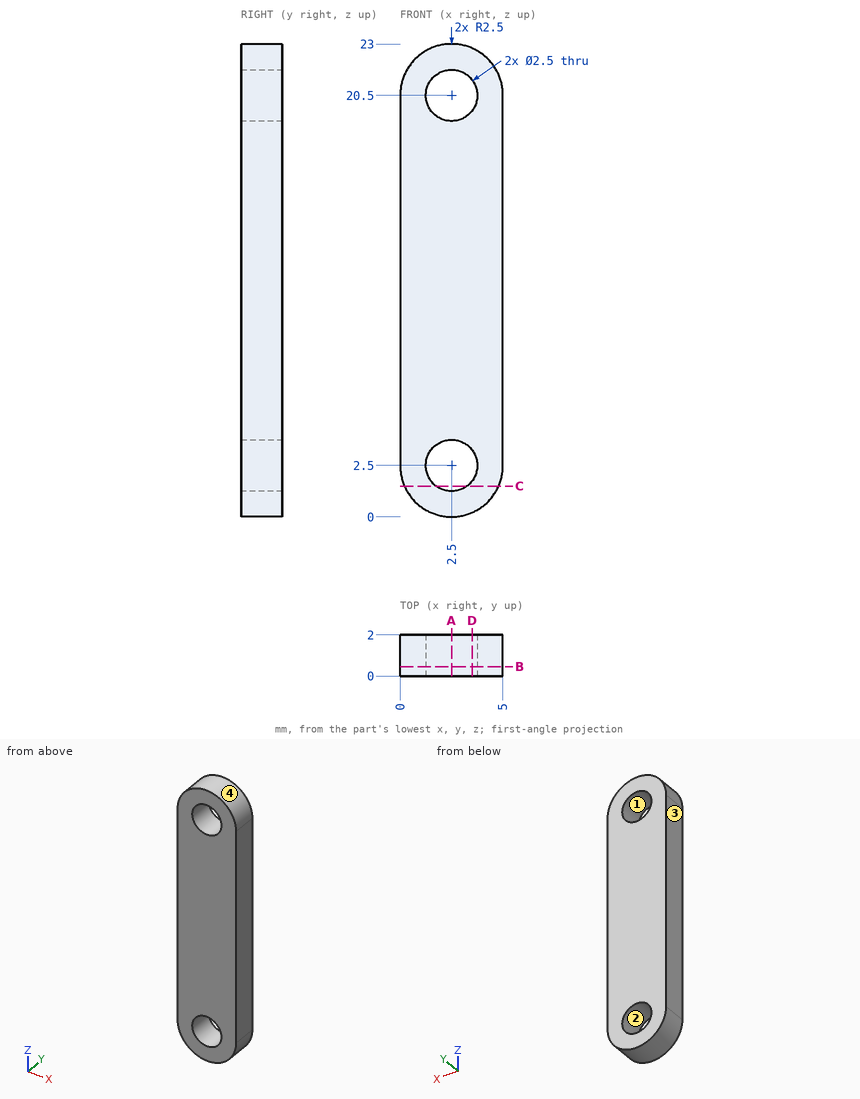
Geometry: see drawing. Coordinates: mm, zero at the bounding-box minimum. Give positions to 0.01 mm unless a question says otherwise; leave off trailing zeros. Loops run counter-clockwise (first coordinate to the right, second up) from the corner with the lowest first, then second, coordinate; pieces in that order, holes last. Notation, with made-up numbers: (55.25, 33.25) - (96.25, 33.25) arc R20 cw to (96.25, 61.25) - close; hole circle Ø9 at (50, -20.75). An arc over 180 degrees is marked (long way). One line per question, with ' | ' between items. Start each with the question number.
(1) Ray query, line 1 (X direction, y = 0.75, z = 20.5); line 2 (Z direction, x = 2.6, y = 0.2); line 3 (Z direction, x = 3.35, y = 0.5). Return the intervals inside material, ascending. Write a range as from..to.
(2) Section query C-C on z = 1.5. Return loops of the section in (x, y).
(3) Contact query for a flat-ended pin moving along its axis: pin 1 (3 mm diameter, centred on x = 2.5, z = 2.5, fed in from -Y). Output: stop coordinate, or through.
(4) Section query D-D on x = 3.5. Return loops of the section in (y, z).
(5) Pull-direction query (X, two-part tool) for the marked faces 1, 2, 3 and 4; classes: released by +X, released by -X, zero draft, split by the parting line, or undercut.
(6) Section query B-B on y = 0.45. Return loops of the section in (x, z), then the cut area to 3 significant figures.
(7) Section query A-A on x = 2.5. Return loops of the section in (y, z), then the cut area to 3 significant figures.
The answers:
1) line 1: 0..1.25, 3.75..5 | line 2: 0..1.25, 3.75..19.25, 21.75..23 | line 3: 0.15..1.58, 3.42..19.58, 21.42..22.85
2) outline: (0.21, 0) - (1.75, 0) - (1.75, 2) - (0.21, 2) - close; (3.25, 0) - (4.79, 0) - (4.79, 2) - (3.25, 2) - close
3) pin 1: y = 0
4) outline: (0, 0.21) - (2, 0.21) - (2, 1.75) - (0, 1.75) - close; (0, 3.25) - (2, 3.25) - (2, 19.75) - (0, 19.75) - close; (0, 21.25) - (2, 21.25) - (2, 22.79) - (0, 22.79) - close
5) face 1: undercut | face 2: undercut | face 3: released by -X | face 4: split by the parting line
6) outline: (0, 2.5) arc R2.5 ccw to (5, 2.5) - (5, 20.5) arc R2.5 ccw to (0, 20.5) - close; hole circle Ø2.5 at (2.5, 2.5); hole circle Ø2.5 at (2.5, 20.5) | area: 99.8 mm2
7) outline: (0, 0) - (2, 0) - (2, 1.25) - (0, 1.25) - close; (0, 3.75) - (2, 3.75) - (2, 19.25) - (0, 19.25) - close; (0, 21.75) - (2, 21.75) - (2, 23) - (0, 23) - close | area: 36.0 mm2
